```python
from build123d import *

# Parameters (mm, degrees)
BOSS_EXTRUDE1_DEPTH  = 2.9
SOLENOID_PLACEMENT_W = 37.4
SOLENOID_PLACEMENT_H = 63.8
CUT_EXTRUDE1_DEPTH   = 103.571487266
CUT_EXTRUDE2_DEPTH   = 103.571487266
SKETCH3_R            = 12
CUT_EXTRUDE3_DEPTH   = 98.286484159
SKETCH4_R            = 2.25
CUT_EXTRUDE4_DEPTH   = 98.416066437


with BuildPart() as part:
    # Sketch1 → Boss-Extrude1 (new body)
    with BuildSketch(Plane(origin=(0, 0, 0), x_dir=(1, 0, 0), z_dir=(0, 1, 0))):
        with BuildLine():
            ThreePointArc((33.29110537, -64.404598464), (0, 72.5), (-33.29110537, -64.404598464))
            ThreePointArc((-33.29110537, -64.404598464), (0, -44.989799638), (33.29110537, -64.404598464))
        make_face()
    extrude(amount=BOSS_EXTRUDE1_DEPTH)

    # solenoid placement → Cut-Extrude1 (cut, through all)
    with BuildSketch(Plane(origin=(0, 2.9, 0), x_dir=(1, 0, 0), z_dir=(0, 1, 0))):
        with Locations((0, -3.8)):
            Rectangle(SOLENOID_PLACEMENT_W, SOLENOID_PLACEMENT_H)
    extrude(amount=-CUT_EXTRUDE1_DEPTH, mode=Mode.SUBTRACT)

    # Sketch2 → Cut-Extrude2 (cut, through all)
    with BuildSketch(Plane(origin=(0, 2.9, 0), x_dir=(1, 0, 0), z_dir=(0, 1, 0))):
        with BuildLine():
            Line((-34.63, -32.5), (-22.83, -32.5))
            Line((-22.83, -32.5), (-22.83, 32.5))
            Line((-22.83, 32.5), (-64.807406984, 32.5))
            ThreePointArc((-64.807406984, 32.5), (-72.5, 0), (-64.807406984, -32.5))
            Line((-64.807406984, -32.5), (-34.63, -32.5))
        make_face()
        with BuildLine():
            Line((34.63, -32.5), (64.807406984, -32.5))
            ThreePointArc((64.807406984, -32.5), (72.5, 0), (64.807406984, 32.5))
            Line((64.807406984, 32.5), (22.83, 32.5))
            Line((22.83, 32.5), (22.83, -32.5))
            Line((22.83, -32.5), (34.63, -32.5))
        make_face()
    extrude(amount=-CUT_EXTRUDE2_DEPTH, mode=Mode.SUBTRACT)

    # Sketch3 → Cut-Extrude3 (cut, through all)
    with BuildSketch(Plane(origin=(0, 2.9, 0), x_dir=(1, 0, 0), z_dir=(0, 1, 0))):
        with Locations(Location((25, 48, 0), (0, 0, 270))):
            Circle(SKETCH3_R)
        with Locations(Location((-25, 48, 0), (0, 0, 270))):
            Circle(SKETCH3_R)
    extrude(amount=-CUT_EXTRUDE3_DEPTH, mode=Mode.SUBTRACT)

    # Sketch4 → Cut-Extrude4 (cut, through all)
    with BuildSketch(Plane(origin=(0, 5.8, 0), x_dir=(1, 0, 0), z_dir=(0, 1, 0))):
        with Locations(Location((35, -50, 0), (0, 0, 270))):
            Circle(SKETCH4_R)
        with Locations(Location((-35, -50, 0), (0, 0, 270))):
            Circle(SKETCH4_R)
        with Locations(Location((-50, 40, 0), (0, 0, 270))):
            Circle(SKETCH4_R)
        with Locations(Location((50, 40, 0), (0, 0, 270))):
            Circle(SKETCH4_R)
    extrude(amount=-CUT_EXTRUDE4_DEPTH, mode=Mode.SUBTRACT)


solid = part.part
```
Verification items for the finished model (mm, model axes). A direction names the side the tool comes from. Coordinates: 2 decimals unless noted, no trailing zeros. Loops run counter-clockwise (first coordinate to the right, second up) from the corner with the lowest first, then second, coordinate; pieces in that order, holes last. Notation, with made-up numbers: (38, -1.5) - (57, -1.5) arc R13 cw to (57, 21.5) - close; hole circle Ø9 at (-34.75, -3.5). An arc over 180 degrees is marked (long way). Put each result on its own line as item: value.
Item 1: Gauge pin test, flat ends, axial feed: pin 1 Ø2.5 at (x, z) = (50, -40) entering from +Y; pin 2 Ø0.9 at (y, z) = (1, -7.5) entering from -X; pin 3 Ø1.4 at (x, y) = (-5.5, 1.5) entering from +Z; pin 4 Ø1.4 at (y, z) = (1, 0.5) entering from +X. Record the tip position at first contact, or that the pin passes through.
Conclusion:
pin 1: passes through
pin 2: stops at x = -22.83
pin 3: stops at z = 45.5
pin 4: stops at x = 22.83
Item 2: Section check D-D (x = 35). Enter the section's corners in (y, z), then the cut area to 3 significant figures.
Conclusion:
outline: (0, -63.49) - (2.9, -63.49) - (2.9, -54.63) - (0, -54.63) - close; (0, -41.37) - (2.9, -41.37) - (2.9, -32.5) - (0, -32.5) - close; (0, 32.5) - (2.9, 32.5) - (2.9, 47.75) - (0, 47.75) - close; (0, 52.25) - (2.9, 52.25) - (2.9, 63.49) - (0, 63.49) - close
area: 128 mm2
Item 3: Draft check along Z on faces 1 (the face through (51.35, 1.43, 51.18)), 2 (the face through (36.52, 1.47, 48.34)), 3 (the face through (-1, 2.9, -35)). Enter one of: pulls with the +Z half, pulls with the -Z half, needs draft (parallel to the pull), parting line crosses it, or undercut.
Conclusion:
face 1: pulls with the +Z half
face 2: undercut
face 3: needs draft
Item 4: Section check C-C (y = 1.8). Enter the section's corners in (x, z).
Conclusion:
outline: (-64.81, -32.5) arc R72.5 ccw to (64.81, -32.5) - (22.83, -32.5) - (22.83, 32.5) - (64.81, 32.5) arc R72.5 ccw to (33.29, 64.4) arc R38.25 cw to (-33.29, 64.4) arc R72.5 ccw to (-64.81, 32.5) - (-22.83, 32.5) - (-22.83, -32.5) - close; hole circle Ø4.5 at (-50, -40); hole circle Ø4.5 at (-35, 50); hole circle Ø24 at (-25, -48); hole (-18.7, -28.1) - (18.7, -28.1) - (18.7, 35.7) - (-18.7, 35.7) - close; hole circle Ø24 at (25, -48); hole circle Ø4.5 at (35, 50); hole circle Ø4.5 at (50, -40)
Item 5: Section check A-A (x = -50). Enter the section's corners in (y, z).
Conclusion:
outline: (0, -52.5) - (2.9, -52.5) - (2.9, -42.25) - (0, -42.25) - close; (0, -37.75) - (2.9, -37.75) - (2.9, -32.5) - (0, -32.5) - close; (0, 32.5) - (2.9, 32.5) - (2.9, 52.5) - (0, 52.5) - close
Item 6: Section check B-B (z = -12). Enter the section's corners in (x, y), then the cut area to 3 significant figures.
Conclusion:
outline: (-22.83, 0) - (-18.7, 0) - (-18.7, 2.9) - (-22.83, 2.9) - close; (18.7, 0) - (22.83, 0) - (22.83, 2.9) - (18.7, 2.9) - close
area: 24.0 mm2
Item 7: Set-up check for faces 4 (the face through (-44, 1, -32.5)), 5 (the face through (22.83, 1, 0)), 6 (the face through (-18.7, 1, 4)): record each of +Z, -Z, +X, -X, +Y, -Y from which the full face is reachable in a straight line by a thin tool's end or side.
Conclusion:
face 4: -X, +Y, -Y
face 5: +X, +Y, -Y
face 6: +Y, -Y
Item 8: Scan lines: line 1 along X through (y, z) = (0.35, -8.5); line 2 along X through (y, z) = (2.6, -58); line 3 along X through (y, z) = (2.25, -48). Record each from-to range of solid material in increasing order.
Conclusion:
line 1: x = -22.83 to -18.7, 18.7 to 22.83
line 2: x = -43.5 to -31.63, -18.37 to 18.37, 31.63 to 43.5
line 3: x = -54.33 to -37, -13 to 13, 37 to 54.33
